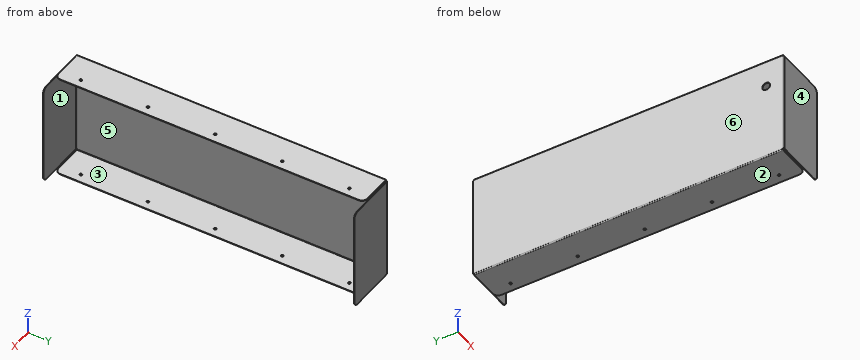
from build123d import *

# Parameters (mm, degrees)
BASE_FLANGE1_DEPTH           = 144
EDGE_FLANGE1_DEPTH           = 872
EDGE_FLANGE1_BEND_DEPTH      = 872
F_7_0_7_DIAMETER_HOLE1_D     = 7
F_7_0_7_DIAMETER_HOLE1_DEPTH = 1.5
FILLET1_R                    = 15
CUT_EXTRUDE1_DEPTH           = 487.946095579


# Sheet-metal steps are written as plain solids
with BuildPart() as part:
    # Sketch1 → Base-Flange1 (new, symmetric)
    with BuildSketch(Plane.XY):
        with BuildLine():
            Line((147, 438), (1.5, 438))
            ThreePointArc((1.5, 438), (0.439339828, 437.560660172), (0, 436.5))
            Line((0, 436.5), (0, -436.5))
            ThreePointArc((0, -436.5), (0.439339828, -437.560660172), (1.5, -438))
            Line((1.5, -438), (147, -438))
            Line((147, -438), (147, -439.5))
            Line((147, -439.5), (1.5, -439.5))
            ThreePointArc((1.5, -439.5), (-0.621320344, -438.621320344), (-1.5, -436.5))
            Line((-1.5, -436.5), (-1.5, 436.5))
            ThreePointArc((-1.5, 436.5), (-0.621320344, 438.621320344), (1.5, 439.5))
            Line((1.5, 439.5), (147, 439.5))
            Line((147, 439.5), (147, 438))
        make_face()
    extrude(amount=BASE_FLANGE1_DEPTH, both=True)

    # Edge-Flange1 section (across the edge) → Edge-Flange1 (add)
    with BuildSketch(Plane(origin=(0, 436, 146.5), x_dir=(0, 0, -1), z_dir=(0, -1, 0))):
        with BuildLine():
            Line((-1.5, 1.5), (-1.5, 98.5))
            Line((-1.5, 98.5), (0, 98.5))
            Line((0, 98.5), (0, 1.5))
            ThreePointArc((0, 1.5), (0.439339828, 0.439339828), (1.5, 0))
            Line((1.5, 0), (2.5, 0))
            Line((2.5, 0), (2.5, -1.5))
            Line((2.5, -1.5), (1.5, -1.5))
            ThreePointArc((1.5, -1.5), (-0.621320344, -0.621320344), (-1.5, 1.5))
        make_face()
    extrude(amount=EDGE_FLANGE1_DEPTH)

    # Edge-Flange1 section 2 (across the edge) → Edge-Flange1 bend (add)
    with BuildSketch(Plane(origin=(0, -436, -146.5), x_dir=(0, 0, 1), z_dir=(0, 1, 0))):
        with BuildLine():
            Line((-1.5, 1.5), (-1.5, 98.5))
            Line((-1.5, 98.5), (0, 98.5))
            Line((0, 98.5), (0, 1.5))
            ThreePointArc((0, 1.5), (0.439339828, 0.439339828), (1.5, 0))
            Line((1.5, 0), (2.5, 0))
            Line((2.5, 0), (2.5, -1.5))
            Line((2.5, -1.5), (1.5, -1.5))
            ThreePointArc((1.5, -1.5), (-0.621320344, -0.621320344), (-1.5, 1.5))
        make_face()
    extrude(amount=EDGE_FLANGE1_BEND_DEPTH)

    # Ø7.0 (7) Diameter Hole1
    with Locations(Plane(origin=(0, 0, 146.5), x_dir=(-1, 0, 0), z_dir=(0, 0, -1))):
        with Locations((-74.25, 379.5), (-74.25, 190), (-74.25, 0.5), (-74.25, -189), (-74.25, -378.5)):
            f_7_0_7_diameter_hole1 = Hole(F_7_0_7_DIAMETER_HOLE1_D / 2, depth=F_7_0_7_DIAMETER_HOLE1_DEPTH)

    # Mirror1: Ø7.0 (7) Diameter Hole1 across plane
    add(f_7_0_7_diameter_hole1.mirror(Plane.XY), mode=Mode.SUBTRACT)

    # Fillet1
    fillet1_edges = [part.edges().sort_by_distance(p)[0] for p in [
        (147, 438.75, -144),
        (147, -438.75, -144),
        (147, 438.75, 144),
        (98.5, 436, 147.25),
        (98.5, -436, 147.25),
        (98.5, -436, -147.25),
        (98.5, 436, -147.25),
        (147, -438.75, 144),
    ]]
    fillet(fillet1_edges, radius=FILLET1_R)

    # Sketch14 → Cut-Extrude1 (cut, through all)
    with BuildSketch(Plane.ZY.offset(1.5)):
        with BuildLine():
            Line((80.5, -392.778719262), (80.5, -386.221280738))
            ThreePointArc((80.5, -386.221280738), (70, -378.5), (59.5, -386.221280738))
            Line((59.5, -386.221280738), (59.5, -392.778719262))
            ThreePointArc((59.5, -392.778719262), (70, -400.5), (80.5, -392.778719262))
        make_face()
    extrude(amount=-CUT_EXTRUDE1_DEPTH, mode=Mode.SUBTRACT)


solid = part.part
The model under review builds one solid part; all positions refer to its coordinate system, in mm. Face numbers are marked on the shaded views. A direction names the side the tool comes from. Coordinates: 2 decimals unless noted, no trailing zeros. Write each loop counter-clockwise with the first axis right and the second up, starting at its lowest first coordinate (ties: lowest second). Pieces come first, ordered by that corner, then holes. Notation, with made-up numbers: M 34.5,35 L 64.5,35 A32 cw 64.5,61 Z; hole C -29,14.25 d1. An arc over 180 degrees is marked long. Put each result on its own line as item: value.
1) Draft analysis for pull direction Y (two halves, no side actions). For the marked faces 4, 5 and 6, state which applies: released by +Y, released by -Y, zero draft, split by the parting line, or undercut.
Computed:
face 4: released by -Y
face 5: undercut
face 6: zero draft
2) Add section C-C on x = 37. Give the boundary of the cut face in (y, z), then the cut area to 3 significant figures.
Computed:
outline: M -439.5,-144 L -438,-144 L -438,144 L -439.5,144 Z; M -436,-148 L 436,-148 L 436,-146.5 L -436,-146.5 Z; M -436,146.5 L 436,146.5 L 436,148 L -436,148 Z; M 438,-144 L 439.5,-144 L 439.5,144 L 438,144 Z
area: 3,480 mm2
3) Add section D-D on y = 167. Give the boundary of the cut face in (x, z), then the cut area to 3 significant figures.
Computed:
outline: M -1.5,-145 A3 ccw 1.5,-148 L 98.5,-148 L 98.5,-146.5 L 1.5,-146.5 A1.5 cw 0,-145 L 0,145 A1.5 cw 1.5,146.5 L 98.5,146.5 L 98.5,148 L 1.5,148 A3 ccw -1.5,145 Z
area: 737 mm2
4) Add section B-B on z = 48. Give the boundary of the cut face in (x, y).
Computed:
outline: M -1.5,-436.5 A3 ccw 1.5,-439.5 L 147,-439.5 L 147,-438 L 1.5,-438 A1.5 cw 0,-436.5 L 0,436.5 A1.5 cw 1.5,438 L 147,438 L 147,439.5 L 1.5,439.5 A3 ccw -1.5,436.5 Z
5) Clearance check with flat-ended pins moving along their axes: pin 1 Ø11 at (x, y) = (74.25, 379.5) entering from -Z; pin 2 Ø1.2 at (y, z) = (-198, 147) entering from +X; pin 3 Ø4 at (x, y) = (74.25, -189) entering from +Z; pin 4 Ø1.5 at (y, z) = (-278.5, 9) entering from +X. State where each tip first meets the part, or that it passes through.
Computed:
pin 1: stops at z = -148
pin 2: stops at x = 98.5
pin 3: passes through
pin 4: stops at x = 0
6) For the marked faces 1, 2 and 3, list the 3-axis set-ups (+Z, -Z, +X, -X, +Y, -Y) from which the entire face can be reached by the end or side of a thin tool; tool diameter is ignored.
Computed:
face 1: +Z, -Z, +X
face 2: -Z, +X, -X, +Y, -Y
face 3: +X, +Y, -Y
7) Add section A-A on x = 109.5. Give the boundary of the cut face in (y, z), then the cut area to 3 significant figures.
Computed:
outline: M -439.5,-144 L -438,-144 L -438,144 L -439.5,144 Z; M 438,-144 L 439.5,-144 L 439.5,144 L 438,144 Z
area: 864 mm2
8) Wall thickness on probe 1 along Y at (x, z) = (74.25, 147.25); probe 2 along Y at (x, z) = (84, -50.5); probe 3 along Z at (x, y) = (49.5, -64.5): over which ranges is each line inside the solid? List them lowest first. Write a range as [from, to].
Computed:
probe 1: y = [-436, -382], [-375, -192.5], [-185.5, -3], [4, 186.5], [193.5, 376], [383, 436]
probe 2: y = [-439.5, -438], [438, 439.5]
probe 3: z = [-148, -146.5], [146.5, 148]
